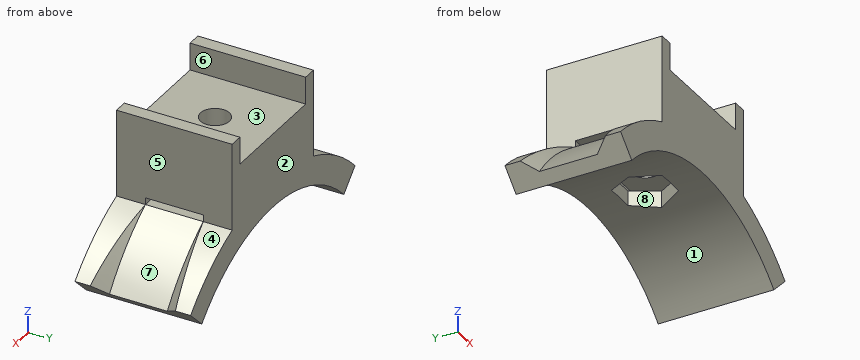
from build123d import *

# Parameters (mm, degrees)
BOSS_EXTRUDE1_DEPTH     = 25.4
SKETCH2_W               = 1.5
SKETCH2_H               = 12.7
CUT_EXTRUDE1_DEPTH      = 81.888878871
CUT_EXTRUDE2_DEPTH      = 12.7
SKETCH6_R               = 3.175
CUT_EXTRUDE4_DEPTH      = 50.335811816
CUT_EXTRUDE5_DEPTH      = 4.365625
CUT_EXTRUDE5_DEPTH_BACK = 47.366407345


with BuildPart() as part:
    # Sketch1 → Boss-Extrude1 (new body)
    with BuildSketch(Plane(origin=(0, 0, 0), x_dir=(1, 0, 0), z_dir=(0, 1, 0))):
        with BuildLine():
            Line((-12.7, -54.385), (12.7, -54.385))
            Line((12.7, -54.385), (12.7, -60.385))
            Line((12.7, -60.385), (15.7, -60.385))
            Line((15.7, -60.385), (15.7, -41.210678228))
            ThreePointArc((15.7, -41.210678228), (24.31025853, -36.794311112), (31.75, -30.606331044))
            Line((31.75, -30.606331044), (27.430272109, -26.442204372))
            ThreePointArc((27.430272109, -26.442204372), (0, -38.1), (-27.430272109, -26.442204372))
            Line((-27.430272109, -26.442204372), (-31.75, -30.606331044))
            ThreePointArc((-31.75, -30.606331044), (-24.31025853, -36.794311112), (-15.7, -41.210678228))
            Line((-15.7, -41.210678228), (-15.7, -60.385))
            Line((-15.7, -60.385), (-12.7, -60.385))
            Line((-12.7, -60.385), (-12.7, -54.385))
        make_face()
    extrude(amount=BOSS_EXTRUDE1_DEPTH)

    # Sketch2 → Cut-Extrude1 (cut, through all)
    with BuildSketch(Plane(origin=(15.7, 0, 0), x_dir=(0, 0, -1), z_dir=(1, 0, 0))):
        with Locations((-41.960678228, 12.7)):
            Rectangle(SKETCH2_W, SKETCH2_H)
    extrude(amount=-CUT_EXTRUDE1_DEPTH, mode=Mode.SUBTRACT)

    # Sketch3 → Cut-Extrude2 (cut)
    with BuildSketch(Plane(origin=(0, 6.35, 0), x_dir=(1, 0, 0), z_dir=(0, 1, 0))):
        with BuildLine():
            Line((31.75, -30.606331044), (29.590136054, -28.524267708))
            ThreePointArc((29.590136054, -28.524267708), (23.300825781, -35.585451028), (15.7, -41.210678228))
            ThreePointArc((15.7, -41.210678228), (24.31025853, -36.794311112), (31.75, -30.606331044))
        make_face()
    cut_extrude2 = extrude(amount=CUT_EXTRUDE2_DEPTH, mode=Mode.SUBTRACT)

    # Mirror1: Cut-Extrude2 across plane
    add(cut_extrude2.mirror(Plane(origin=(0, 0, 0), x_dir=(0, 0, 1), z_dir=(1, 0, 0))), mode=Mode.SUBTRACT)

    # Sketch6 → Cut-Extrude4 (cut, through all)
    with BuildSketch(Plane.XY.offset(54.385)):
        with Locations((0, 12.7)):
            Circle(SKETCH6_R)
    extrude(amount=-CUT_EXTRUDE4_DEPTH, mode=Mode.SUBTRACT)

    # Sketch7 → Cut-Extrude5 (cut, two sides: drawn at the far end of the back side and taken through both)
    with BuildSketch(Plane.XY.offset(38.1).offset(-CUT_EXTRUDE5_DEPTH_BACK)):
        Polygon((6.415804866, 12.7), (3.207902433, 18.25625), (-3.207902433, 18.25625), (-6.415804866, 12.7), (-3.207902433, 7.14375), (3.207902433, 7.14375), align=None)
    extrude(amount=CUT_EXTRUDE5_DEPTH + CUT_EXTRUDE5_DEPTH_BACK, mode=Mode.SUBTRACT)

    # Cut-Sweep1: sweep along a path in Sketch9
    with BuildLine(Plane.XZ.offset(-19.05)) as cut_sweep1_path:
        ThreePointArc((29.590136054, 28.524267708), (23.300825781, 35.585451028), (15.7, 41.210678228))
    # Sketch8 → Cut-Sweep1 (sweep, cut)
    with BuildSketch(Plane(origin=(0, 0, 0), x_dir=(-0.7199546485260769, 0, -0.6940211121181352), z_dir=(0.6940211121181352, 0, -0.7199546485260769))):
        Polygon((-44.1, 19.05), (-41.1, 19.05), (-44.1, 22.05), align=None)
    cut_sweep1 = sweep(path=cut_sweep1_path.line, mode=Mode.SUBTRACT)

    # Mirror2: Cut-Sweep1 across plane
    add(cut_sweep1.mirror(Plane.ZX.offset(12.7)), mode=Mode.SUBTRACT)

    # Mirror3: Cut-Sweep1 across plane
    add(cut_sweep1.mirror(Plane(origin=(0, 0, 0), x_dir=(0, 0, 1), z_dir=(1, 0, 0))), mode=Mode.SUBTRACT)

    # Mirror3 copy 1: sweep along a path in Mirror3 copy 1 path
    with BuildLine(Plane(origin=(0, 6.35, 0), x_dir=(-1, 0, 0), z_dir=(0, 1, 0))) as mirror3_copy_1_path:
        ThreePointArc((29.590136054, 28.524267708), (23.300825781, 35.585451028), (15.7, 41.210678228))
    # Mirror3 copy 1 sketch → Mirror3 copy 1 (sweep, cut)
    with BuildSketch(Plane(origin=(0, 25.4, 0), x_dir=(0.7199546485260769, 0, -0.6940211121181352), z_dir=(-0.6940211121181352, 0, -0.7199546485260769))):
        Polygon((-44.1, 19.05), (-41.1, 19.05), (-44.1, 22.05), align=None)
    sweep(path=mirror3_copy_1_path.line, mode=Mode.SUBTRACT)


solid = part.part
CAD build for the part. Positions are in the model's coordinates, mm. Face numbers are marked on the shaded views. A direction names the side the tool comes from. Coordinates: 2 decimals unless noted, no trailing zeros. Loops run counter-clockwise (first coordinate to the right, second up) from the corner with the lowest first, then second, coordinate; pieces in that order, holes last. Notation, with made-up numbers: (-18.5, 30.5) - (20.5, 30.5) arc R19 cw to (20.5, 53.5) - close; hole circle Ø9 at (6.25, 51.5). An arc over 180 degrees is marked (long way). Write item = value, one per line. Start each with the question number.
Q1. Which spindle directions (+Z, -Z, +X, -X, +Y, -Y) get a long thin tool onto all of the face, cutting with end or side? Do the marked faces 5, 6, 7 and 8. Say none if no direction does.
Q2. Cut at B-B, the plane z = 53. List the corners of the cut face in (x, y) (3 decimals), then the cut area to 3 significant figures.
Q3. Cut at C-C, the plane x = -9. List the corners of the cut face in (y, z) (3 decimals).
Q4. Drill centre lines: L1, parallel to Y at x = 0, z = 46.5 (3 decimals); L2, parallel to X at y = 12.5, z = 51; L3, parallel to X at y = 6.5, z = 51.5. Where is each one in solid material? Low to high.
Q5. Cut at D-D, the plane y = 14.75. List the corners of the cut face in (x, z) (3 decimals).
Q6. Cut at A-A, the plane x = 0. List the corners of the cut face in (y, z) (3 decimals), then the cut area to 3 significant figures.
Q7. Pull direction X, two halves, no side cores. Call the marked faces 1, 2, 3 and 4: pulls with the +X half, pulls with the -X half, needs draft (parallel to the pull), parting line crosses it, or undercut.
Q8. Flat gauge pins, fed straight in: pin 1 Ø8 at (y, z) = (21.5, 51) entering from +X; pin 2 Ø4 at (x, y) = (4.5, 11) entering from -Z; pin 3 Ø4 at (y, z) = (20.5, 51.5) entering from -X. Where does each tip first touch, or does it go through?
Computed:
q1.face_5 = +Z, +X, +Y, -Y
q1.face_6 = +Z, +Y, -Y
q1.face_7 = +Z, +X
q1.face_8 = -Z
q2.outline = (-15.7, 0) - (15.7, 0) - (15.7, 25.4) - (-15.7, 25.4) - close; hole circle Ø6.35 at (0, 12.7)
q2.area = 766 mm²
q3.outline = (0, 37.022) - (25.4, 37.022) - (25.4, 54.385) - (0, 54.385) - close; hole (6.35, 41.211) - (19.05, 41.211) - (19.05, 42.711) - (6.35, 42.711) - close
q4.L1 = 0 to 9.525, 15.875 to 25.4
q4.L2 = -15.7 to -3.17, 3.17 to 15.7
q4.L3 = -15.7 to 15.7
q5.outline = (-29.59, 28.524) - (-27.43, 26.442) arc R38.1 cw to (-5.232, 37.739) - (-5.232, 41.211) - (-15.7, 41.211) arc R45.978 ccw to start; (-15.7, 42.711) - (-2.424, 42.711) - (-2.424, 54.385) - (-12.7, 54.385) - (-12.7, 60.385) - (-15.7, 60.385) - close; (2.424, 42.711) - (15.7, 42.711) - (15.7, 60.385) - (12.7, 60.385) - (12.7, 54.385) - (2.424, 54.385) - close; (5.232, 37.739) arc R38.1 cw to (27.43, 26.442) - (29.59, 28.524) arc R45.978 ccw to (15.7, 41.211) - (5.232, 41.211) - close
q6.outline = (0, 38.1) - (7.144, 38.1) - (7.144, 41.211) - (6.35, 41.211) - (6.35, 42.711) - (9.525, 42.711) - (9.525, 54.385) - (0, 54.385) - close; (15.875, 42.711) - (19.05, 42.711) - (19.05, 41.211) - (18.256, 41.211) - (18.256, 38.1) - (25.4, 38.1) - (25.4, 54.385) - (15.875, 54.385) - close
q6.area = 286 mm²
q7.face_1 = undercut
q7.face_2 = needs draft
q7.face_3 = undercut
q7.face_4 = pulls with the +X half
q8.pin_1 = 15.7
q8.pin_2 = 37.54
q8.pin_3 = -15.7
